Geometry check sheet. Reference: the model listing, model coordinates, mm. Face numbers are marked on the shaded views. Coordinates: 2 decimals unless noted, no trailing zeros. Order: outer loops, then holes, each group sorted by start corner. A loop starts at its lowest first (then second) coordinate and runs counter-clockwise, first axis right, second up. Notation, with made-up numbers: (41.5, -37) - (45.5, -37) arc R27 cw to (45.5, -17) - close; hole circle Ø10 at (22, 39). An arc over 180 degrees is marked (long way). Put each result on its own line as item: value.
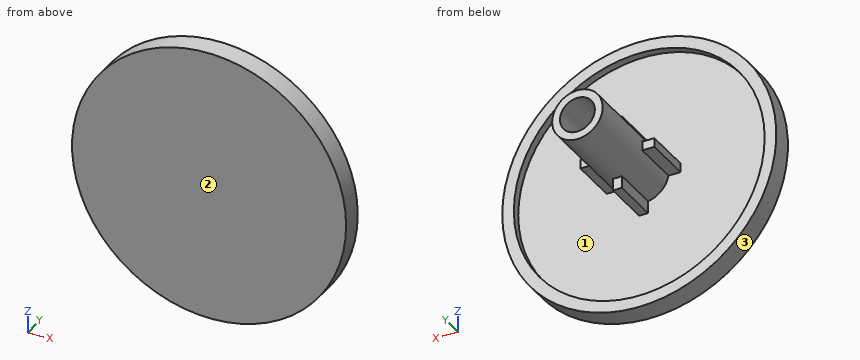
from build123d import *

# Parameters (mm, degrees)
SKETCH1_R           = 13.1699
BOSS_EXTRUDE1_DEPTH = 1.27
SKETCH2_R           = 13.1699
SKETCH2_R_2         = 12.0523
BOSS_EXTRUDE2_DEPTH = 0.762
SKETCH3_R           = 2.4257
BOSS_EXTRUDE3_DEPTH = 11.5443
SKETCH6_W           = 7.112
SKETCH6_H           = 5.842
BOSS_EXTRUDE4_DEPTH = 0.4318
SKETCH7_W           = 7.112
SKETCH7_H           = 5.842
BOSS_EXTRUDE5_DEPTH = 0.4318
SKETCH4_R           = 1.6764
CUT_EXTRUDE1_DEPTH  = 11.5443


with BuildPart() as part:
    # Sketch1 → Boss-Extrude1 (new body)
    with BuildSketch(Plane(origin=(0, 0, 0), x_dir=(1, 0, 0), z_dir=(0, 1, 0))):
        Circle(SKETCH1_R)
    extrude(amount=BOSS_EXTRUDE1_DEPTH)

    # Sketch2 → Boss-Extrude2 (add)
    with BuildSketch(Plane(origin=(0, 1.27, 0), x_dir=(1, 0, 0), z_dir=(0, 1, 0))):
        Circle(SKETCH2_R)
        Circle(SKETCH2_R_2, mode=Mode.SUBTRACT)
    extrude(amount=BOSS_EXTRUDE2_DEPTH)

    # Sketch3 → Boss-Extrude3 (add)
    with BuildSketch(Plane(origin=(0, 1.27, 0), x_dir=(1, 0, 0), z_dir=(0, 1, 0))):
        Circle(SKETCH3_R)
    extrude(amount=BOSS_EXTRUDE3_DEPTH)

    # Sketch6 → Boss-Extrude4 (add, symmetric)
    with BuildSketch(Plane.XY):
        with Locations((0, 2.921)):
            Rectangle(SKETCH6_W, SKETCH6_H)
    extrude(amount=BOSS_EXTRUDE4_DEPTH, both=True)

    # Sketch7 → Boss-Extrude5 (add, symmetric)
    with BuildSketch(Plane(origin=(0, 0, 0), x_dir=(0, 0, -1), z_dir=(1, 0, 0))):
        with Locations((0, 2.921)):
            Rectangle(SKETCH7_W, SKETCH7_H)
    extrude(amount=BOSS_EXTRUDE5_DEPTH, both=True)

    # Sketch4 → Cut-Extrude1 (cut)
    with BuildSketch(Plane(origin=(0, 12.8143, 0), x_dir=(1, 0, 0), z_dir=(0, 1, 0))):
        Circle(SKETCH4_R)
    extrude(amount=-CUT_EXTRUDE1_DEPTH, mode=Mode.SUBTRACT)


solid = part.part
Q1. Draft check along X on the marked faces 1, 2 and 3. Enter one of: pulls with the +X half, pulls with the -X half, needs draft (parallel to the pull), parting line crosses it, or undercut.
Answer block:
face 1: undercut
face 2: needs draft
face 3: parting line crosses it
Q2. Section check B-B on z = 0. Record the boundary of the cut face in (x, y), then the cut area to 3 significant figures.
Answer block:
outline: (-13.17, 0) - (13.17, 0) - (13.17, 2.03) - (12.05, 2.03) - (12.05, 1.27) - (3.56, 1.27) - (3.56, 5.84) - (2.43, 5.84) - (2.43, 12.81) - (1.68, 12.81) - (1.68, 1.27) - (-1.68, 1.27) - (-1.68, 12.81) - (-2.43, 12.81) - (-2.43, 5.84) - (-3.56, 5.84) - (-3.56, 1.27) - (-12.05, 1.27) - (-12.05, 2.03) - (-13.17, 2.03) - close
area: 62.8 mm^2
Q3. Section check A-A on y = 3. Record the boundary of the cut face in (x, z), then the cut area to 3 significant figures.
Answer block:
outline: (-3.56, -0.43) - (-2.39, -0.43) arc R2.43 ccw to (-0.43, -2.39) - (-0.43, -3.56) - (0.43, -3.56) - (0.43, -2.39) arc R2.43 ccw to (2.39, -0.43) - (3.56, -0.43) - (3.56, 0.43) - (2.39, 0.43) arc R2.43 ccw to (0.43, 2.39) - (0.43, 3.56) - (-0.43, 3.56) - (-0.43, 2.39) arc R2.43 ccw to (-2.39, 0.43) - (-3.56, 0.43) - close; hole circle Ø3.35 at (0, 0)
area: 13.6 mm^2
Q4. Section check D-D on x = -4.25. Record the boundary of the cut face in (y, z).
Answer block:
outline: (0, -12.47) - (2.03, -12.47) - (2.03, -11.28) - (1.27, -11.28) - (1.27, 11.28) - (2.03, 11.28) - (2.03, 12.47) - (0, 12.47) - close
Q5. Thickness scan on L1, parallel to Z at x = 0, y = 1.8; L2, parallel to Z at x = 0, y = 9. Record the ranges inside material, lowest first. Write a range as [from, to].
Answer block:
L1: z = [-13.17, -12.05], [-3.56, -1.68], [1.68, 3.56], [12.05, 13.17]
L2: z = [-2.43, -1.68], [1.68, 2.43]
Q6. Section check C-C on x = 0. Record the boundary of the cut face in (y, z).
Answer block:
outline: (0, -13.17) - (2.03, -13.17) - (2.03, -12.05) - (1.27, -12.05) - (1.27, -3.56) - (5.84, -3.56) - (5.84, -2.43) - (12.81, -2.43) - (12.81, -1.68) - (1.27, -1.68) - (1.27, 1.68) - (12.81, 1.68) - (12.81, 2.43) - (5.84, 2.43) - (5.84, 3.56) - (1.27, 3.56) - (1.27, 12.05) - (2.03, 12.05) - (2.03, 13.17) - (0, 13.17) - close
Q7. Depth check by flat-ended pin: pin 1 Ø0.7 at (y, z) = (3.5, 0) entering from -X; pin 2 Ø2 at (x, y) = (-8, 2.5) entering from +Z; pin 3 Ø0.6 at (y, z) = (4, 3) entering from -X. Enter the tip coordinate at first touch or a pass-through.
Answer block:
pin 1: stops at x = -3.56
pin 2: stops at z = 11.08
pin 3: stops at x = -0.43
